Here's how the part is built. I have some questions about the finished solid (model axes, mm). Face numbers are marked on the shaded views. A direction names the side the tool comes from. Round coordinates to 2 decimals unless told otherwise and drop trailing zeros. Write each loop counter-clockwise with the first axis right and the second up, starting at its lowest first coordinate (ties: lowest second). Pieces come first, ordered by that corner, then holes. Notation, with made-up numbers: (9, -28.5) -> (55, -28.5) arc R15 ccw to (55, -18.5) -> close; hole circle Ø9 at (37.25, 1.25). An arc over 180 degrees is marked (long way). Put each result on its own line as item: value. Start each with the question number.
1. Suppose I cut it at B-B (z = 17). Please give me the cut outline in (x, y).
2. We'd pull the mould along Y, two halves only. Please class the marked faces 1, 2 and 3: +Y half, -Y half, draft (parallel to the pull), parting line (faces both ways), or undercut.
3. Suppose I cut it at D-D (y = -20.25). Please give me the cut outline in (x, z), then the cut area to 3 significant figures.
4. Suppose I cut it at A-A (y = -15). Please give me the cut outline in (x, z).
5. Which directions (+Z, -Z, +X, -X, +Y, -Y) give clear straight access to the entire face, cutting with the end or side of a thin tool? Please do the marked faces 4, 5 and 6.
6. I need wall thicknesses on probe 1 along Z at (x, y) = (1.5, -15); probe 2 along Z at (x, y) = (-14, -2.5); probe 3 along X at (y, z) = (-7, 26.5). Which ranges of each line are inside material? Lowest first, please. Write a range as from..to.
7. Suppose I cut it at C-C (x = 2.5). Please give me the cut outline in (y, z).
8. For pin 1 (8 mm diameter, centred on y = -4.5, z = 8, fed in from +X); pin 2 (3 mm diameter, centred on x = -10, y = -5.5, fed in from +Z); pin 3 (4 mm diameter, centred on x = -2.5, y = -4.5, fed in from +Z), each with a flat end and sliding along its axis, tell me the tip position at first contact or that it passes through.
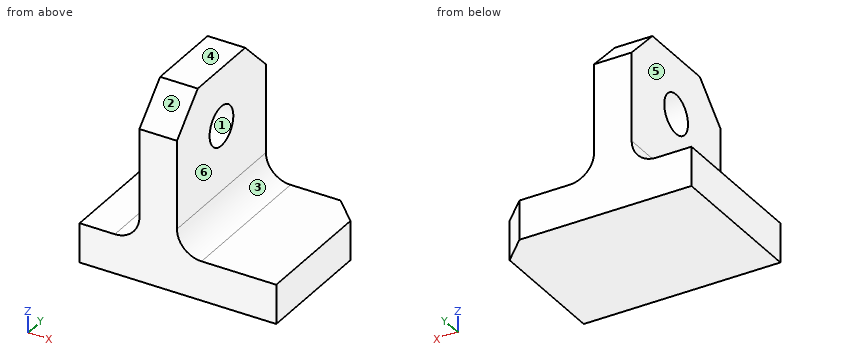
```python
from build123d import *

# Parameters (mm, degrees)
SKETCH_1_W          = 7.64
SKETCH_1_H          = 30
EXTRUDE_1_DEPTH     = 30
SKETCH_2_W          = 40
SKETCH_2_H          = 29.999999992
EXTRUDE_2_DEPTH     = 8
FILLET_1_R          = 5
CHAMFER_1_SIZE      = 7
SKETCH_3_R          = 4
CUT_EXTRUDE_1_DEPTH = 51.742711323
CHAMFER_2_SIZE      = 5


with BuildPart() as part:
    # Эскиз1 → Вытянуть1 (new body)
    with BuildSketch(Plane.XY):
        with Locations((-0.195638171, -15)):
            Rectangle(SKETCH_1_W, SKETCH_1_H)
    extrude(amount=EXTRUDE_1_DEPTH)

    # Эскиз2 → Вытянуть2 (add)
    with BuildSketch(Plane(origin=(0, 0, 0), x_dir=(-1, 0, 0), z_dir=(0, 0, -1))):
        with Locations((-3.82, -14.999999996)):
            Rectangle(SKETCH_2_W, SKETCH_2_H)
    extrude(amount=EXTRUDE_2_DEPTH)

    # Скругление1
    fillet_1_edges = [part.edges().sort_by_distance(p)[0] for p in [
        (-4.015638171, -15, 0),
        (3.624361829, -15, 0),
    ]]
    fillet(fillet_1_edges, radius=FILLET_1_R)

    # Фаска1
    chamfer_1_edges = [part.edges().sort_by_distance(p)[0] for p in [
        (-0.195638171, -30, 30),
        (-0.195638171, 0, 30),
    ]]
    chamfer(chamfer_1_edges, length=CHAMFER_1_SIZE)

    # Эскиз3 → Вырез-Вытянуть1 (cut, through all)
    with BuildSketch(Plane.ZY.offset(4.015638171)):
        with Locations(Location((18.228841689, -15, 0), (0, 0, 270))):
            Circle(SKETCH_3_R)
    extrude(amount=-CUT_EXTRUDE_1_DEPTH, mode=Mode.SUBTRACT)

    # Фаска2
    chamfer_2_edges = [part.edges().sort_by_distance(p)[0] for p in [
        (23.82, 0, -4),
    ]]
    chamfer(chamfer_2_edges, length=CHAMFER_2_SIZE)


solid = part.part
```
Verdict:
1. outline: (-4.02, -30) -> (3.62, -30) -> (3.62, -18.81) -> (-4.02, -18.81) -> close; (-4.02, -11.19) -> (3.62, -11.19) -> (3.62, 0) -> (-4.02, 0) -> close
2. face 1: undercut
2. face 2: -Y half
2. face 3: draft
3. outline: (-16.18, -8) -> (23.82, -8) -> (23.82, 0) -> (8.62, 0) arc R5 cw to (3.62, 5) -> (3.62, 30) -> (-4.02, 30) -> (-4.02, 5) arc R5 cw to (-9.02, 0) -> (-16.18, 0) -> close
3. area: 560 mm^2
4. outline: (-16.18, -8) -> (23.82, -8) -> (23.82, 0) -> (8.62, 0) arc R5 cw to (3.62, 5) -> (3.62, 14.23) -> (-4.02, 14.23) -> (-4.02, 5) arc R5 cw to (-9.02, 0) -> (-16.18, 0) -> close; (-4.02, 22.23) -> (3.62, 22.23) -> (3.62, 30) -> (-4.02, 30) -> close
5. face 4: +Z, +X, -X, +Y, -Y
5. face 5: +Z, -X, +Y, -Y
5. face 6: +Z, +X, +Y, -Y
6. probe 1: z = -8..14.23, 22.23..30
6. probe 2: z = -8..0
6. probe 3: x = -4.02..3.62
7. outline: (-30, -8) -> (0, -8) -> (0, 23) -> (-7, 30) -> (-23, 30) -> (-30, 23) -> close; hole circle Ø8 at (-15, 18.23)
8. pin 1: stops at x = 3.73
8. pin 2: stops at z = 0.03
8. pin 3: stops at z = 29.5
